from build123d import *

# Parameters (mm, degrees)
SKETCH_1_W          = 20
SKETCH_1_H          = 20
EXTRUDE_1_DEPTH     = 430
EXTRUDE_1_2_DEPTH   = 430
EXTRUDE_1_3_DEPTH   = 430
EXTRUDE_1_4_DEPTH   = 430
SKETCH_2_W          = 20
SKETCH_2_H          = 20
EXTRUDE_2_DEPTH     = 260
SKETCH_3_W          = 20
SKETCH_3_H          = 20
EXTRUDE_3_DEPTH     = 160
SKETCH_5_W          = 20
SKETCH_5_H          = 20
EXTRUDE_4_DEPTH     = 261
SKETCH_6_W          = 20
SKETCH_6_H          = 20
EXTRUDE_6_DEPTH     = 160
SKETCH_7_R          = 5
CUT_EXTRUDE_2_DEPTH = 41


with BuildPart() as part:
    # Sketch 1 → Extrude 1 (new body)
    with BuildSketch(Plane.XY):
        with Locations((-140, 90)):
            Rectangle(SKETCH_1_W, SKETCH_1_H)
    extrude(amount=EXTRUDE_1_DEPTH)



with BuildPart() as body_2:
    # Sketch 1 → Extrude 1 2 (new body)
    with BuildSketch(Plane.XY):
        with Locations((-140, -90)):
            Rectangle(SKETCH_1_W, SKETCH_1_H)
    extrude(amount=EXTRUDE_1_2_DEPTH)


with BuildPart() as body_3:
    # Sketch 1 → Extrude 1 3 (new body)
    with BuildSketch(Plane.XY):
        with Locations((140, -90)):
            Rectangle(SKETCH_1_W, SKETCH_1_H)
    extrude(amount=EXTRUDE_1_3_DEPTH)


with BuildPart() as body_4:
    # Sketch 1 → Extrude 1 4 (new body)
    with BuildSketch(Plane.XY):
        with Locations((140, 90)):
            Rectangle(SKETCH_1_W, SKETCH_1_H)
    extrude(amount=EXTRUDE_1_4_DEPTH)


with BuildPart() as part_1:
    add(part.part)

    add(body_2.part)  # Extrude 2 merges body 2

    add(body_3.part)  # Extrude 2 merges body 3

    add(body_4.part)  # Extrude 2 merges body 4
    # Sketch 2 → Extrude 2 (add)
    with BuildSketch(Plane(origin=(-130, 0, 0), x_dir=(0, 0, -1), z_dir=(1, 0, 0))):
        with Locations((-10, 90)):
            Rectangle(SKETCH_2_W, SKETCH_2_H)
        with Locations((-10, -90)):
            Rectangle(SKETCH_2_W, SKETCH_2_H)
    extrude(amount=EXTRUDE_2_DEPTH)

    # Sketch 3 → Extrude 3 (add)
    with BuildSketch(Plane(origin=(0, -80, 0), x_dir=(1, 0, 0), z_dir=(0, 1, 0))):
        with Locations((140, -10)):
            Rectangle(SKETCH_3_W, SKETCH_3_H)
        with Locations((-140, -10)):
            Rectangle(SKETCH_3_W, SKETCH_3_H)
    extrude(amount=EXTRUDE_3_DEPTH)

    # Sketch 5 → Extrude 4 (add)
    with BuildSketch(Plane(origin=(-130, 0, 0), x_dir=(0, 0, -1), z_dir=(1, 0, 0))):
        with Locations((-330, 90)):
            Rectangle(SKETCH_5_W, SKETCH_5_H)
        with Locations((-330, -90)):
            Rectangle(SKETCH_5_W, SKETCH_5_H)
    extrude(amount=EXTRUDE_4_DEPTH)

    # Sketch 6 → Extrude 6 (add)
    with BuildSketch(Plane.XZ.offset(-80)):
        with Locations((140, 301.284847627)):
            Rectangle(SKETCH_6_W, SKETCH_6_H)
        with Locations((-140, 301.284847627)):
            Rectangle(SKETCH_6_W, SKETCH_6_H)
    extrude(amount=EXTRUDE_6_DEPTH)

    # Sketch 7 → Cut-Extrude 2 (cut)
    with BuildSketch(Plane.XY.offset(20)):
        with Locations((110, 90)):
            Circle(SKETCH_7_R)
        with Locations((110, -90)):
            Circle(SKETCH_7_R)
        with Locations((-110, -90)):
            Circle(SKETCH_7_R)
        with Locations((-110, 90)):
            Circle(SKETCH_7_R)
    extrude(amount=-CUT_EXTRUDE_2_DEPTH, mode=Mode.SUBTRACT)


solid = part_1.part
Geometry: final body of the model. Coordinates: model frame, mm. A direction names the side the tool comes from. Give positions to 0.01 mm unless a question says otherwise; leave off trailing zeros. Order: outer loops, then holes, each group sorted by start corner. A loop starts at its lowest first (then second) coordinate and runs counter-clockwise, first axis right, second up. Notation, with made-up numbers: (85.25, 54) -> (140.25, 54) arc R16 cw to (140.25, 64) -> close; hole circle Ø8 at (73.5, 70.5). An arc over 180 degrees is marked (long way). Put each result on its own line as item: value.
Q1. Section D-D, the plane y = -90. Return loops of the section in (x, z).
Here are the results:
outline: (-150, 0) -> (-115, 0) -> (-115, 20) -> (-130, 20) -> (-130, 320) -> (130, 320) -> (130, 20) -> (115, 20) -> (115, 0) -> (150, 0) -> (150, 430) -> (130, 430) -> (130, 340) -> (-130, 340) -> (-130, 430) -> (-150, 430) -> close; (-105, 0) -> (105, 0) -> (105, 20) -> (-105, 20) -> close
Q2. Pin query (flat end, axial travel): pin 1 (11.5 mm diameter, centred on x = 110, y = 90, fed in from -Z); pin 2 (16 mm diameter, centred on x = 60, y = -87, fed in from +Z); pin 3 (6 mm diameter, centred on x = -143.5, y = 10, fed in from +Z). Return the tip coordinate at first contact, or that it passes through.
Here are the results:
pin 1: stops at z = 0
pin 2: stops at z = 340
pin 3: stops at z = 311.28
Q3. Section B-B, the plane y = -47. Return loops of the section in (x, z).
Here are the results:
outline: (-150, 0) -> (-130, 0) -> (-130, 20) -> (-150, 20) -> close; (-150, 291.28) -> (-130, 291.28) -> (-130, 311.28) -> (-150, 311.28) -> close; (130, 0) -> (150, 0) -> (150, 20) -> (130, 20) -> close; (130, 291.28) -> (150, 291.28) -> (150, 311.28) -> (130, 311.28) -> close
Q4. Section C-C, the plane x = -110. Return loops of the section in (y, z).
Here are the results:
outline: (-100, 0) -> (-95, 0) -> (-95, 20) -> (-100, 20) -> close; (-100, 320) -> (-80, 320) -> (-80, 340) -> (-100, 340) -> close; (-85, 0) -> (-80, 0) -> (-80, 20) -> (-85, 20) -> close; (80, 0) -> (85, 0) -> (85, 20) -> (80, 20) -> close; (80, 320) -> (100, 320) -> (100, 340) -> (80, 340) -> close; (95, 0) -> (100, 0) -> (100, 20) -> (95, 20) -> close
Q5. Section A-A, the plane x = -19. Return loops of the section in (y, z), then the cut area to 3 significant figures.
Here are the results:
outline: (-100, 0) -> (-80, 0) -> (-80, 20) -> (-100, 20) -> close; (-100, 320) -> (-80, 320) -> (-80, 340) -> (-100, 340) -> close; (80, 0) -> (100, 0) -> (100, 20) -> (80, 20) -> close; (80, 320) -> (100, 320) -> (100, 340) -> (80, 340) -> close
area: 1,600 mm^2
Q6. Reachability of faces 1 (the face through (114.619, -91.915, 10.14)), 2 (the face through (130, -1, 10)), 3 (the face through (-2, -90, 340)), 4 (the face through (-2, -90, 320)) from +Z, -Z, +X, -X, +Y, -Y: full face, straight path, thin tool, end or side. Return the list, or none.
Here are the results:
face 1: -Z
face 2: +Z, -Z
face 3: +Z, +Y, -Y
face 4: +Y, -Y
Q7. Material intervals for L1, parallel to Y at x = 110, z = 4.75; L2, parallel to Z at x = 93, y = 83; L3, parallel to X at y = -65.5, z = 291.5, sorted ascending.
Here are the results:
L1: y = -100 to -95, -85 to -80, 80 to 85, 95 to 100
L2: z = 0 to 20, 320 to 340
L3: x = -150 to -130, 130 to 150
Q8. Draft query along Y for faces 5 (the face through (140, 1, 291.285)), 6 (the face through (-2, 87, 0)). Return one class per face: released by +Y, released by -Y, zero draft, split by the parting line, or undercut.
Here are the results:
face 5: undercut
face 6: zero draft
